from build123d import *

# Parameters (mm, degrees)
SKETCH1_W           = 304.8
SKETCH1_H           = 152.4
BOSS_EXTRUDE1_DEPTH = 6.35
CUT_EXTRUDE1_REACH  = 8.35
SKETCH2_R           = 12.7
SKETCH2_R_2         = 4.7625


with BuildPart() as part:
    # Sketch1 → Boss-Extrude1 (new body)
    with BuildSketch(Plane(origin=(0, 0, 0), x_dir=(1, 0, 0), z_dir=(0, 1, 0))):
        with Locations((152.4, 76.2)):
            Rectangle(SKETCH1_W, SKETCH1_H)
    extrude(amount=BOSS_EXTRUDE1_DEPTH)

    # Sketch2 → Cut-Extrude1 (cut, up to next)
    with BuildSketch(Plane(origin=(0, 6.35, 0), x_dir=(-1, 0, 0), z_dir=(0, 1, 0)), mode=Mode.PRIVATE) as cut_extrude1_sk1:
        with Locations((-25.4, -19.05)):
            Circle(SKETCH2_R)
    cut_extrude1_tool1 = extrude(cut_extrude1_sk1.sketch, amount=-CUT_EXTRUDE1_REACH, mode=Mode.PRIVATE) & part.part
    add(cut_extrude1_tool1.solids().sort_by_distance((25.4, 6.35, -19.05))[0], mode=Mode.SUBTRACT)
    # Sketch2 → Cut-Extrude1 (cut, up to next)
    with BuildSketch(Plane(origin=(0, 6.35, 0), x_dir=(-1, 0, 0), z_dir=(0, 1, 0)), mode=Mode.PRIVATE) as cut_extrude1_sk2:
        with Locations((-293.6875, -133.35)):
            Circle(SKETCH2_R_2)
    cut_extrude1_tool2 = extrude(cut_extrude1_sk2.sketch, amount=-CUT_EXTRUDE1_REACH, mode=Mode.PRIVATE) & part.part
    add(cut_extrude1_tool2.solids().sort_by_distance((293.6875, 6.35, -133.35))[0], mode=Mode.SUBTRACT)
    # Sketch2 → Cut-Extrude1 (cut, up to next)
    with BuildSketch(Plane(origin=(0, 6.35, 0), x_dir=(-1, 0, 0), z_dir=(0, 1, 0)), mode=Mode.PRIVATE) as cut_extrude1_sk3:
        with Locations((-11.1125, -133.35)):
            Circle(SKETCH2_R_2)
    cut_extrude1_tool3 = extrude(cut_extrude1_sk3.sketch, amount=-CUT_EXTRUDE1_REACH, mode=Mode.PRIVATE) & part.part
    add(cut_extrude1_tool3.solids().sort_by_distance((11.1125, 6.35, -133.35))[0], mode=Mode.SUBTRACT)
    # Sketch2 → Cut-Extrude1 (cut, up to next)
    with BuildSketch(Plane(origin=(0, 6.35, 0), x_dir=(-1, 0, 0), z_dir=(0, 1, 0)), mode=Mode.PRIVATE) as cut_extrude1_sk4:
        with Locations((-11.1125, -73.025)):
            Circle(SKETCH2_R_2)
    cut_extrude1_tool4 = extrude(cut_extrude1_sk4.sketch, amount=-CUT_EXTRUDE1_REACH, mode=Mode.PRIVATE) & part.part
    add(cut_extrude1_tool4.solids().sort_by_distance((11.1125, 6.35, -73.025))[0], mode=Mode.SUBTRACT)
    # Sketch2 → Cut-Extrude1 (cut, up to next)
    with BuildSketch(Plane(origin=(0, 6.35, 0), x_dir=(-1, 0, 0), z_dir=(0, 1, 0)), mode=Mode.PRIVATE) as cut_extrude1_sk5:
        with Locations((-293.6875, -73.025)):
            Circle(SKETCH2_R_2)
    cut_extrude1_tool5 = extrude(cut_extrude1_sk5.sketch, amount=-CUT_EXTRUDE1_REACH, mode=Mode.PRIVATE) & part.part
    add(cut_extrude1_tool5.solids().sort_by_distance((293.6875, 6.35, -73.025))[0], mode=Mode.SUBTRACT)
    # Sketch2 → Cut-Extrude1 (cut, up to next)
    with BuildSketch(Plane(origin=(0, 6.35, 0), x_dir=(-1, 0, 0), z_dir=(0, 1, 0)), mode=Mode.PRIVATE) as cut_extrude1_sk6:
        with Locations((-279.4, -19.05)):
            Circle(SKETCH2_R)
    cut_extrude1_tool6 = extrude(cut_extrude1_sk6.sketch, amount=-CUT_EXTRUDE1_REACH, mode=Mode.PRIVATE) & part.part
    add(cut_extrude1_tool6.solids().sort_by_distance((279.4, 6.35, -19.05))[0], mode=Mode.SUBTRACT)


solid = part.part
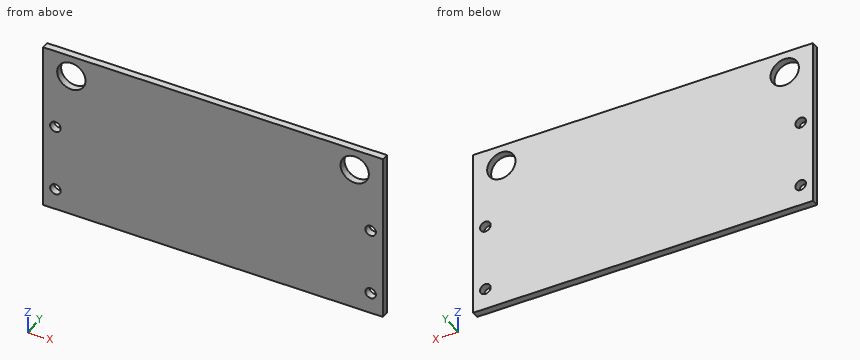
Could you check a few things on this model? Use its own coordinates, in mm. Round coordinates to 2 decimals unless told otherwise and drop trailing zeros. Order: outer loops, then holes, each group sorted by start corner. A loop starts at its lowest first (then second) coordinate and runs counter-clockwise, first axis right, second up.
Q1. Imagine slicing it at C-C, the plane z = -133.35. List the corners of the cut face in (x, y) for me (3 decimals).
Geometry says:
outline: (0, 0) - (6.35, 0) - (6.35, 6.35) - (0, 6.35) - close; (15.875, 0) - (288.925, 0) - (288.925, 6.35) - (15.875, 6.35) - close; (298.45, 0) - (304.8, 0) - (304.8, 6.35) - (298.45, 6.35) - close
Q2. Please list where these lines run through material, in increasing order: probe 1 along X at (y, z) = (5.75, -23); probe 2 along X at (y, z) = (2.5, -75).
Geometry says:
probe 1: x = 0 to 13.33, 37.47 to 267.33, 291.47 to 304.8
probe 2: x = 0 to 6.78, 15.45 to 289.35, 298.02 to 304.8
Q3. I'm going to push flat-ended pins straight in: P1, Ø5.5, axis at x = 293.69, z = -133.35, coming from the -Y side; P2, Ø12, axis at x = 241, z = -125.5, coming from the -Y side. Where does each tip first touch, or does it pass through?
Geometry says:
P1: passes through
P2: stops at y = 0
Q4. Imagine slicing it at D-D, the plane y = 4.25. State how many separate pieces and enclosed holes the cut face has, then the cut area to 3 significant figures.
Geometry says:
separate pieces: 1
enclosed holes: 6
area: 45,200 mm2
Q5. Imagine slicing it at B-B, the plane x = 279.4. List the corners of the cut face in (y, z) for me, then the cut area to 3 significant figures.
Geometry says:
outline: (0, -152.4) - (6.35, -152.4) - (6.35, -31.75) - (0, -31.75) - close; (0, -6.35) - (6.35, -6.35) - (6.35, 0) - (0, 0) - close
area: 806 mm2
Q6. Imagine slicing it at A-A, the plane z = -19.05. List the corners of the cut face in (x, y) for me, then the cut area to 3 significant figures.
Geometry says:
outline: (0, 0) - (12.7, 0) - (12.7, 6.35) - (0, 6.35) - close; (38.1, 0) - (266.7, 0) - (266.7, 6.35) - (38.1, 6.35) - close; (292.1, 0) - (304.8, 0) - (304.8, 6.35) - (292.1, 6.35) - close
area: 1,610 mm2
